Verification items for the finished model (mm, model axes). Face numbers are marked on the shaded views. A direction names the side the tool comes from. Round coordinates to 2 decimals unless told otherwise and drop trailing zeros. Order: outer loops, then holes, each group sorted by start corner. A loop starts at its lowest first (then second) coordinate and runs counter-clockwise, first axis right, second up. Notation, with made-up numbers: M 84,-34.5 L 130,-34.5 A25 ccw 130,-13.5 Z; hole C 86,-2 d9. An arc over 180 degrees is marked long. Answer as a JSON object with one key per item and string values. Group by question number.
```python
from build123d import *

# Parameters (mm, degrees)
F1_DEPTH  = 2
F2_R      = 4.725
F2_R_2    = 4.225
F3_DEPTH  = 9
F4_W      = 20
F4_H      = 10
F5_DEPTH  = 9
F6_R      = 2.475
F7_DEPTH  = 10
F9_R      = 2.125
F10_DEPTH = 10
F12_R     = 5.5
F12_R_2   = 4.725
F13_DEPTH = 0.5


with BuildPart() as f1:
    # F0 (on Front) → F1 (new body)
    with BuildSketch(Plane.XZ):
        with BuildLine():
            ThreePointArc((-10, 8.3066238629), (0, 13), (10, 8.3066238629))
            Line((10, 8.3066238629), (10, 25))
            Line((10, 25), (-10, 25))
            Line((-10, 25), (-10, 8.3066238629))
        make_face()
        with BuildLine():
            Line((10, 0), (10, 8.3066238629))
            ThreePointArc((10, 8.3066238629), (0, 13), (-10, 8.3066238629))
            Line((-10, 8.3066238629), (-10, 0))
            ThreePointArc((-10, 0), (0, 10), (10, 0))
        make_face()
        with BuildLine():
            ThreePointArc((-10, 0), (0, -10), (10, 0))
            Line((10, 0), (5, 0))
            ThreePointArc((5, 0), (0, -5), (-5, 0))
            Line((-5, 0), (-10, 0))
        make_face()
        with BuildLine():
            Line((5, 0), (10, 0))
            ThreePointArc((10, 0), (0, 10), (-10, 0))
            Line((-10, 0), (-5, 0))
            ThreePointArc((-5, 0), (0, 5), (5, 0))
        make_face()
        with BuildLine():
            Line((4.5, 0), (5, 0))
            ThreePointArc((5, 0), (0, 5), (-5, 0))
            Line((-5, 0), (-4.5, 0))
            ThreePointArc((-4.5, 0), (0, 4.5), (4.5, 0))
        make_face()
        with BuildLine():
            ThreePointArc((-5, 0), (0, -5), (5, 0))
            Line((5, 0), (4.5, 0))
            ThreePointArc((4.5, 0), (0, -4.5), (-4.5, 0))
            Line((-4.5, 0), (-5, 0))
        make_face()
    extrude(amount=F1_DEPTH)

    # F2 (on face) → F3 (join)
    with BuildSketch(Plane.XZ.offset(2)):
        Circle(F2_R)
        Circle(F2_R_2, mode=Mode.SUBTRACT)
    extrude(amount=F3_DEPTH)

    # F4 (on face) → F5 (join)
    with BuildSketch(Plane.XZ.offset(2)):
        with Locations((0, 20)):
            Rectangle(F4_W, F4_H)
    extrude(amount=F5_DEPTH)


with BuildPart() as f7:
    # F6 (on face) → F7 (new body)
    with BuildSketch(Plane.XY.offset(25)):
        with Locations((0, -5.5)):
            Circle(F6_R)
    extrude(amount=-F7_DEPTH)


with BuildPart() as f1_1:
    add(f1.part)

    # F8: cut F7
    add(f7.part, mode=Mode.SUBTRACT)


with BuildPart() as f10:
    # F9 (on face) → F10 (new body)
    with BuildSketch(Plane.XZ.offset(11)):
        with Locations((-6, 20)):
            Circle(F9_R)
    extrude(amount=-F10_DEPTH)


with BuildPart() as f10b:
    # F9 (on face) → F10, piece 2 (new body)
    with BuildSketch(Plane.XZ.offset(11)):
        with Locations((6, 20)):
            Circle(F9_R)
    extrude(amount=-F10_DEPTH)


with BuildPart() as f1_2:
    add(f1_1.part)

    # F11: cut F10b, F10
    add(f10b.part, mode=Mode.SUBTRACT)
    add(f10.part, mode=Mode.SUBTRACT)

    # F12 (on face) → F13 (join)
    with BuildSketch(Plane.XZ.offset(2)):
        Circle(F12_R)
        Circle(F12_R_2, mode=Mode.SUBTRACT)
    extrude(amount=F13_DEPTH)


solid = f1_2.part
```
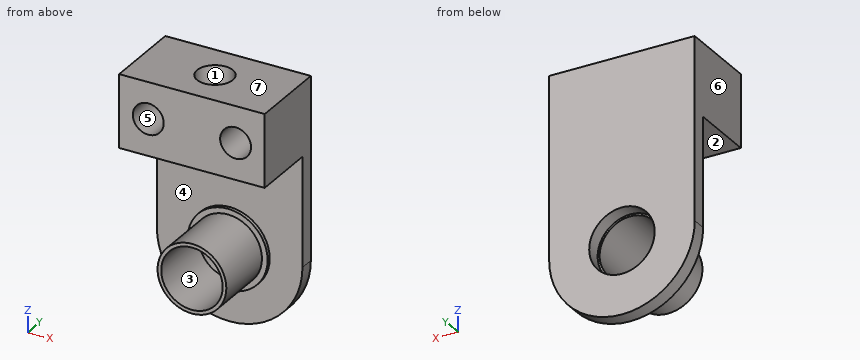
Q1. Cross-section at B-B, the plane y = -5.5. Record the cut outline in (x, z) (3 decimals), then the cut area to 3 significant figures.
Q2. Gauge pin test, flat ends, axial feed: pin 1 Ø12 at (x, z) = (-0.5, 18.5) entering from +Y; pin 2 Ø4.5 at (x, y) = (0, -5.5) entering from -Z (3 decimals); pin 3 Ø4.5 at (x, y) = (3.5, -8) entering from -Z; pin 4 Ø1.5 at (x, z) = (6, 7.5) entering from -Y. Record the tip position at first contact, or that the pin passes through.
Q3. Thickness scan on line 1 (Z direction, x = 0, y = -9.5) (3 decimals); line 2 (X direction, y = -7, z = 20.5); line 3 (Z direction, x = 6, y = -6) (3 decimals). Record the ranges inside material, lowest first. Write a range as from..to.
Q4. Cross-section at A-A, the plane x = 0. Record the cut outline in (y, z) (3 decimals), then the cut area to 3 significant figures.
Q5. Cross-section at C-C, the plane z = 20. Record the cut outline in (x, y) (3 decimals).
Q6. Release check for a two-part mould opening along X. For the marked faces 5, 6 and 7 record: released by +X, released by -X, zero draft, split by the parting line, or undercut.
Q7. Cross-section at D-D, the plane y = -8.5. Record the cut outline in (x, z) (3 decimals), then the cut area to 3 significant figures.
Q8. Tool access check on the marked faces 1, 2, 3 and 4. Record the directions out of +Z, -Z, +X, -X, +Y, -Y that give a thin tool (end or side, any length) a straight path to the whole face; none if there is none.
Conclusion:
{
 "1": {"outline": "M -10,15 L -2.475,15 L -2.475,25 L -10,25 Z; C 0,0 d9.45; M 2.475,15 L 10,15 L 10,25 L 2.475,25 Z; hole C -6,20 d4.25; hole C 0,0 d8.45; hole C 6,20 d4.25", "area": "136 mm2"},
 "2": {"pin 1": "y = 0", "pin 2": "z = -4.725", "pin 3": "z = -4.56", "pin 4": "y = -2"},
 "3": {"line 1": "-4.725..-4.225, 4.225..4.725, 15..25", "line 2": "-10..-8.07, -3.93..-1.97, 1.97..3.93, 8.07..10", "line 3": "15..17.875, 22.125..25"},
 "4": {"outline": "M -11,-4.725 L -2.5,-4.725 L -2.5,-5.5 L -2,-5.5 L -2,-10 L 0,-10 L 0,-4.5 L -2,-4.5 L -2,-4.225 L -11,-4.225 Z; M -11,4.225 L -2,4.225 L -2,4.5 L 0,4.5 L 0,25 L -3.025,25 L -3.025,15 L -2,15 L -2,5.5 L -2.5,5.5 L -2.5,4.725 L -11,4.725 Z; M -11,15 L -7.975,15 L -7.975,25 L -11,25 Z", "area": "102 mm2"},
 "5": {"outline": "M -10,-11 L -8.125,-11 L -8.125,-1 L -3.875,-1 L -3.875,-11 L 3.875,-11 L 3.875,-1 L 8.125,-1 L 8.125,-11 L 10,-11 L 10,0 L -10,0 Z; hole C 0,-5.5 d4.95"},
 "6": {"face 5": "undercut", "face 6": "released by -X", "face 7": "zero draft"},
 "7": {"outline": "M -10,15 L 10,15 L 10,25 L -10,25 Z; C 0,0 d9.45; hole C -6,20 d4.25; hole C 0,0 d8.45; hole C 6,20 d4.25", "area": "186 mm2"},
 "8": {"face 1": "+Z", "face 2": "+X, -X, -Y", "face 3": "+Y, -Y", "face 4": "-Y"}
}
